Part model, mm, in its own coordinate system. Face numbers are marked on the shaded views. A direction names the side the tool comes from. Give positions to 0.01 mm unless a question says otherwise; leave off trailing zeros. Write each loop counter-clockwise with the first axis right and the second up, starting at its lowest first coordinate (ties: lowest second). Pieces come first, ordered by that corner, then holes.
Autodesk Fusion 360 part; units mm, degrees
sketch "Sketch1" plane through (0, 0, 0) normal (0, 0, 1) x (1, 0, 0) in component "exercise 2"
  circle A0 centre (0, 0) radius 30
  line L0 (0, 0) -> (129, 0) construction
  circle A1 centre (129, 0) radius 22.5
  line L1 (28.2843, 10) -> (108.8444, 10)
  line L2 (28.2843, -10) -> (108.8444, -10)
  line L3 (-11.547, 20) -> (-23.094, 0)
  line L4 (-23.094, 0) -> (-11.547, -20)
  line L5 (-11.547, -20) -> (11.547, -20)
  line L6 (11.547, -20) -> (23.094, 0)
  line L7 (23.094, 0) -> (11.547, 20)
  line L8 (11.547, 20) -> (-11.547, 20)
  line L9 (140.0205, -14.9103) -> (146.5861, 5.8736)
  line L10 (146.5861, 5.8736) -> (128.8482, 18.5404)
  line L11 (128.8482, 18.5404) -> (111.3201, 5.585)
  line L12 (111.3201, 5.585) -> (118.225, -15.0887)
  line L13 (118.225, -15.0887) -> (140.0205, -14.9103)
  line L14 (64.5, 0) -> (64.5, 50) construction
  line L15 (38.2534, 0) -> (64.5, 0)
  line L16 (43.2534, 0) -> (98.2534, 0) construction
  line L17 (38.2534, 5) -> (98.2534, 5)
  line L18 (38.2534, -5) -> (98.2534, -5)
  arc A2 (38.2534, 5) -> (38.2534, -5) centre (38.2534, 0) ccw
  arc A3 (98.2534, -5) -> (98.2534, 5) centre (98.2534, 0) ccw
  point P0 (129, 0)
  dimension "d1" = 60
  dimension "d2" = 45
  dimension "d3" = 129
  dimension "d6" = 20
  dimension "d7" = 15
  dimension "d8" = 10
  dimension "d9" = 10
  dimension "d10" = 60
extrude "Extrude1" add sketch "Sketch1" along normal mid plane 20 contours A0 | A1 makes body 1 at (27.1662, -12.7278, 3.3333) makes body 2 at (151.3882, -2.2403, -3.3333) in component "exercise 2"
extrude "Extrude2" add sketch "Sketch1" along normal mid plane 10 contours A0 A1 L1 L2 bodies 1 2 in component "exercise 2"
extrude "Extrude3" add sketch "Sketch1" along normal mid plane 4 contours L17 L18 A2 A3 bodies 1 in component "exercise 2"
component "exercise 2" placed x (1, 0, 0) y (0, 1, 0) z (0, 0, 1) at (0, 0, 0)
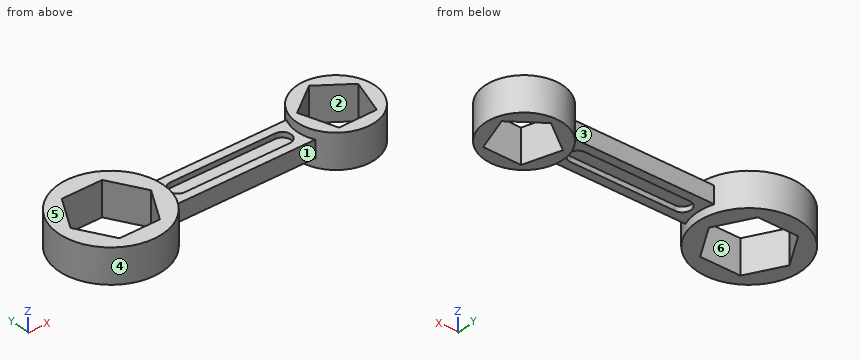
1) Saw through at A-A (x = 0). Write the cut outline in (y, z).
Check result:
outline: (-30, -10) - (-20, -10) - (-20, 10) - (-30, 10) - close; (20, -10) - (30, -10) - (30, 10) - (20, 10) - close
2) Mould opens along Y. For the marked faces 1, 2, 3 and 4 say: +Y half, -Y half, draft (parallel to the pull), parting line (faces both ways), or undercut.
Check result:
face 1: -Y half
face 2: undercut
face 3: +Y half
face 4: parting line
3) Saw through at B-B (y = -13). Write the cut outline in (x, z).
Check result:
outline: (-27.04, -10) - (-15.59, -10) - (-15.59, 10) - (-27.04, 10) - close; (15.59, -10) - (27.04, -10) - (27.04, 10) - (15.59, 10) - close; (110.64, -10) - (117.53, -10) - (117.53, 10) - (110.64, 10) - close; (140.62, -10) - (147.36, -10) - (147.36, 10) - (140.62, 10) - close
4) Drill centre lines: L1, parallel to X at y = -10, z = 8.5; L2, parallel to Y at x = 85, z = -3.5; L3, parallel to X at y = 17.5, z = 4.75. Where is each one in solid material? Low to high.
Check result:
L1: x = -28.28 to -17.32, 17.32 to 28.28, 108.84 to 116.53, 141.57 to 149.16
L2: y = -10 to -5, 5 to 10
L3: x = -24.37 to -12.99, 12.99 to 24.37, 114.86 to 127.44, 130.31 to 143.14
5) Saw through at D-D (x = 113). Write the cut outline in (y, z).
Check result:
outline: (-15.82, -10) - (0.56, -10) - (0.56, 10) - (-15.82, 10) - close; (6.83, -10) - (15.82, -10) - (15.82, 10) - (6.83, 10) - close
6) Saw through at C-C (y = 3). Write the cut outline in (x, z), and give its area (3 significant figures).
Check result:
outline: (-29.85, -10) - (-21.36, -10) - (-21.36, 10) - (-29.85, 10) - close; (21.36, -10) - (29.85, -10) - (29.85, -5) - (34.25, -5) - (34.25, -2) - (102.25, -2) - (102.25, -5) - (106.7, -5) - (106.7, -10) - (112.18, -10) - (112.18, 10) - (106.7, 10) - (106.7, 5) - (102.25, 5) - (102.25, 2) - (34.25, 2) - (34.25, 5) - (29.85, 5) - (29.85, 10) - (21.36, 10) - close; (145.68, -10) - (151.3, -10) - (151.3, 10) - (145.68, 10) - close
area: 922 mm2
7) Flat gauge pins, fed straight in: P1, Ø4, axis at x = 120, z = -4, coming from the -Y side; P2, Ø12, axis at x = 50, z = -2, coming from the -Y side; P3, Ø0.9, axis at x = 57, z = -4, coming from the +Y side. Where does each tip first touch, or does it go through?
Check result:
P1: stops at y = -21.38
P2: stops at y = -10
P3: stops at y = 10
8) 3-axis set-ups, long thin cutter, end or side, ignore diameter. For the marked faces 5 and 6: which of +Z, -Z, +X, -X, +Y, -Y reach the whole face in a straight line?
Check result:
face 5: +Z, +X, -X, +Y, -Y
face 6: +Z, -Z
